Design review of the part built by this model. Coordinates are the model's own, in mm. Face numbers are marked on the shaded views. A direction names the side the tool comes from. Coordinates: 2 decimals unless noted, no trailing zeros. Write each loop counter-clockwise with the first axis right and the second up, starting at its lowest first coordinate (ties: lowest second). Pieces come first, ordered by that corner, then holes.
Q1. Machinability: for the marked faces 1, 2 and 3, which of the approach directions +Z, -Z, +X, -X, +Y, -Y give a long, thin tool a straight path to every point of the face, cutting with its end or side? Answer none if there is none.
Q2. Insertion check: pin 1 (8 mm diameter, centred on x = -8.5, y = 2.5, fed in from +Z); pin 2 (10 mm diameter, centred on x = -3, y = -5.5, fed in from +Z); pin 3 (1.5 mm diameter, centred on x = 5.5, y = 21, fed in from -Z). Each pin has a flat end and moves straight along its axis. Give the tip position at first contact, or say it passes through.
Q3. Take a section at D-D (x = -13). Give the boundary of the cut face in (y, z).
Q4. Take a section at B-B (z = 0). Give the boundary of the cut face in (x, y) (3 decimals).
Q5. For probe 1 along Z at (x, y) = (0, -0.4) (3 decimals); probe 2 along Y at (x, z) = (-5, -9); probe 3 along Y at (x, z) = (-8.5, -15), list the stretches that pass through material, from the lowest coordinate up.
Q6. Take a section at A-A (x = 0). Give the boundary of the cut face in (y, z) (3 decimals).
Q7. Mouldability with a two-part tool opening along Z and no side actions: class the marked faces 4, 5, 6 and 7 as pulls with the +Z half, pulls with the -Z half, needs draft (parallel to the pull), parting line crosses it, or undercut.
Q8. Take a section at C-C (y = -6). Give the boundary of the cut face in (x, z), and give its area (3 significant figures).
```python
from build123d import *

# Parameters (mm, degrees)
SKETCH1_R                = 15.875
BOSS_EXTRUDE1_DEPTH      = 20
SKETCH2_R                = 3.5
BOSS_EXTRUDE2_DEPTH      = 10
BOSS_EXTRUDE2_DEPTH_BACK = 30
SKETCH3_R                = 19.05
SKETCH3_R_2              = 15.875
BOSS_EXTRUDE3_DEPTH      = 21
BOSS_EXTRUDE3_DEPTH_BACK = 1


with BuildPart() as part:
    # Sketch1 → Boss-Extrude1 (new body)
    with BuildSketch(Plane(origin=(0, 0, 0), x_dir=(1, 0, 0), z_dir=(0, 1, 0))):
        Circle(SKETCH1_R)
    extrude(amount=BOSS_EXTRUDE1_DEPTH)

    # Sketch2 → Boss-Extrude2 (add, two sides)
    with BuildSketch(Plane.XZ) as boss_extrude2_sk:
        Circle(SKETCH2_R)
    extrude(amount=BOSS_EXTRUDE2_DEPTH)
    extrude(boss_extrude2_sk.sketch, amount=-BOSS_EXTRUDE2_DEPTH_BACK)

    # Sketch3 → Boss-Extrude3 (add, two sides)
    with BuildSketch(Plane(origin=(0, 0, 0), x_dir=(1, 0, 0), z_dir=(0, 1, 0))) as boss_extrude3_sk:
        Circle(SKETCH3_R)
        Circle(SKETCH3_R_2, mode=Mode.SUBTRACT)
    extrude(amount=BOSS_EXTRUDE3_DEPTH)
    extrude(boss_extrude3_sk.sketch, amount=-BOSS_EXTRUDE3_DEPTH_BACK)


solid = part.part
```
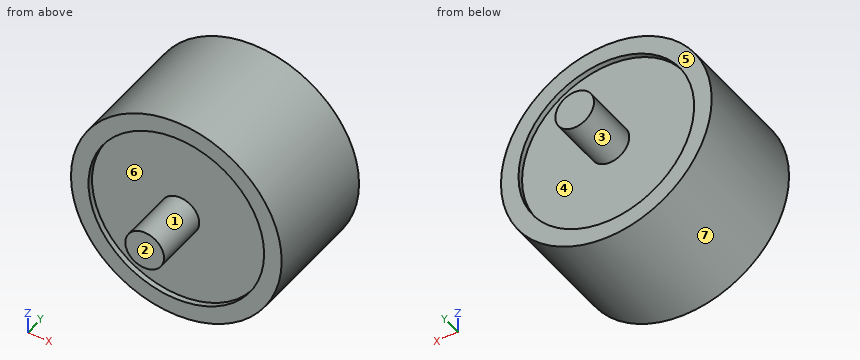
Response:
1. face 1: -Y
1. face 2: +Z, -Z, +X, -X, -Y
1. face 3: +Y
2. pin 1: stops at z = 18.51
2. pin 2: stops at z = 19.03
2. pin 3: stops at z = -18.45
3. outline: (-1, -13.92) - (21, -13.92) - (21, -9.11) - (20, -9.11) - (20, 9.11) - (21, 9.11) - (21, 13.92) - (-1, 13.92) - (-1, 9.11) - (0, 9.11) - (0, -9.11) - (-1, -9.11) - close
4. outline: (-19.05, -1) - (-15.875, -1) - (-15.875, 0) - (-3.5, 0) - (-3.5, -10) - (3.5, -10) - (3.5, 0) - (15.875, 0) - (15.875, -1) - (19.05, -1) - (19.05, 21) - (15.875, 21) - (15.875, 20) - (3.5, 20) - (3.5, 30) - (-3.5, 30) - (-3.5, 20) - (-15.875, 20) - (-15.875, 21) - (-19.05, 21) - close
5. probe 1: z = -19.05 to -15.875, -3.5 to 3.5, 15.875 to 19.05
5. probe 2: y = 0 to 20
5. probe 3: y = -1 to 21
6. outline: (-10, -3.5) - (0, -3.5) - (0, -15.875) - (-1, -15.875) - (-1, -19.05) - (21, -19.05) - (21, -15.875) - (20, -15.875) - (20, -3.5) - (30, -3.5) - (30, 3.5) - (20, 3.5) - (20, 15.875) - (21, 15.875) - (21, 19.05) - (-1, 19.05) - (-1, 15.875) - (0, 15.875) - (0, 3.5) - (-10, 3.5) - close
7. face 4: undercut
7. face 5: needs draft
7. face 6: undercut
7. face 7: parting line crosses it
8. outline: circle Ø7 at (0, 0)
8. area: 38.5 mm2
